Job drawing, mm, ordinate dimensions from the low corner. One solid piece. Coordinates: 2 decimals unless noted, no trailing zeros. Loops run counter-clockwise (first coordinate to the right, second up) from the corner with the lowest first, then second, coordinate; pieces in that order, holes last. Notation, with made-up numbers: M 83,53 L 139,53 A20 ccw 139,89 Z; hole C 24,54.5 d5. An arc over 180 degrees is marked long. Answer as a JSON object with one key per item and string values. Group by question number.
1. Saw through at A-A on z = 33.5. Write the cut outline in (x, y), then the cut area to 3 significant figures.
2. Drill centre lines: L1, parallel to Y at x = 80, z = 94; L2, parallel to Z at x = 13.4, y = 2.7; L3, parallel to Y at x = 30, z = 91. Where is each one in solid material? Low to high.
3. Saw through at D-D on y = 16.25. Write the cut outline in (x, z).
4. Drop flat-ended pins along their axis: pin 1 Ø12 at (x, z) = (66, 29.5) entering from +Y; pin 2 Ø7.5 at (x, y) = (80, 16.25) entering from -Z; pin 3 Ø5.5 at (x, y) = (30, 16.25) entering from -Z. Give the stop position or say it passes through.
5. Saw through at C-C on x = 13.4. Write the cut outline in (y, z).
6. Saw through at B-B on x = 80. Write the cut outline in (y, z), then the cut area to 3 significant figures.
7. Mould opens along Y. For the marked faces 1, 2 and 3 say: released by +Y, released by -Y, zero draft, split by the parting line, or undercut.
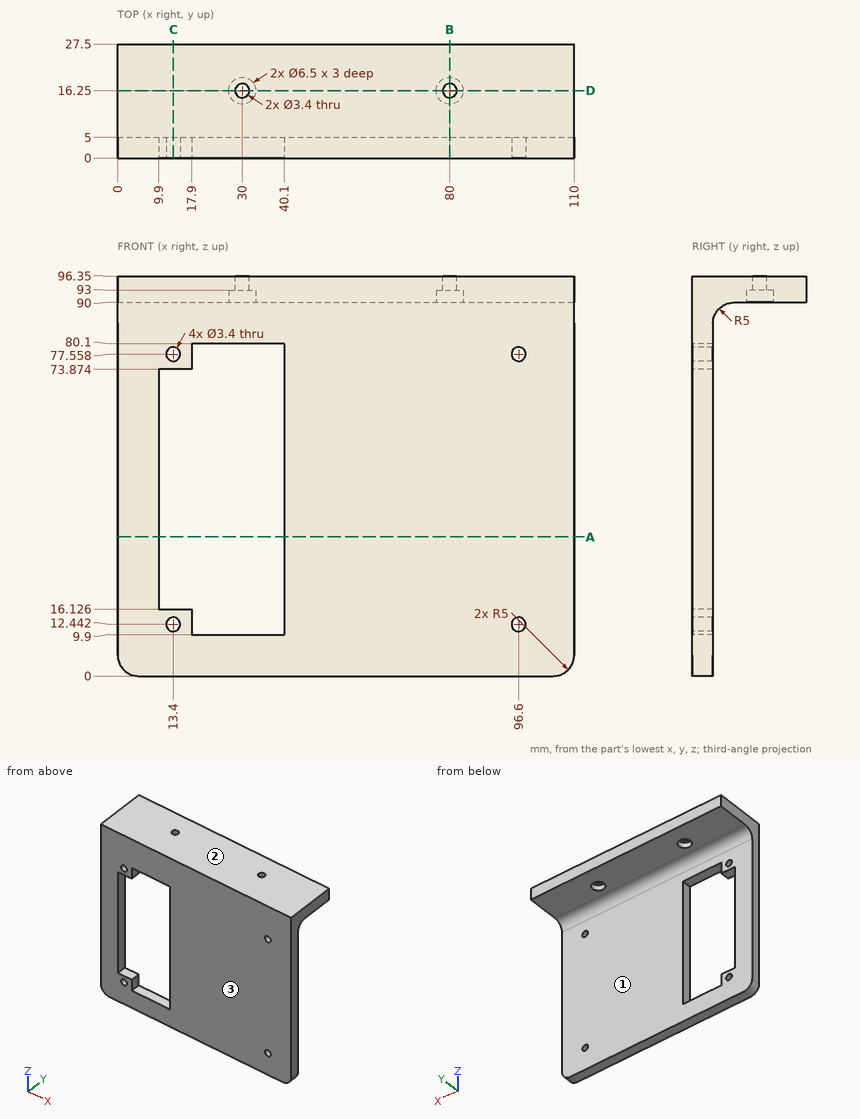
Outcome:
{
 "1": {"outline": "M 0,0 L 9.9,0 L 9.9,5 L 0,5 Z; M 40.1,0 L 110,0 L 110,5 L 40.1,5 Z", "area": "399 mm²"},
 "2": {"L1": "y = 0 to 14.55, 17.95 to 27.5", "L2": "z = 0 to 10.74, 14.14 to 16.13, 73.87 to 75.86, 79.26 to 96.35", "L3": "y = 0 to 13, 19.5 to 27.5"},
 "3": {"outline": "M 0,90 L 26.75,90 L 26.75,93 L 28.3,93 L 28.3,96.35 L 0,96.35 Z; M 31.7,93 L 33.25,93 L 33.25,90 L 76.75,90 L 76.75,93 L 78.3,93 L 78.3,96.35 L 31.7,96.35 Z; M 81.7,93 L 83.25,93 L 83.25,90 L 110,90 L 110,96.35 L 81.7,96.35 Z"},
 "4": {"pin 1": "stops at y = 5", "pin 2": "stops at z = 90", "pin 3": "stops at z = 93"},
 "5": {"outline": "M 0,0 L 5,0 L 5,10.74 L 0,10.74 Z; M 0,14.14 L 5,14.14 L 5,16.13 L 0,16.13 Z; M 0,73.87 L 5,73.87 L 5,75.86 L 0,75.86 Z; M 0,79.26 L 5,79.26 L 5,85 A5 cw 10,90 L 27.5,90 L 27.5,96.35 L 0,96.35 Z"},
 "6": {"outline": "M 0,0 L 5,0 L 5,85 A5 cw 10,90 L 13,90 L 13,93 L 14.55,93 L 14.55,96.35 L 0,96.35 Z; M 17.95,93 L 19.5,93 L 19.5,90 L 27.5,90 L 27.5,96.35 L 17.95,96.35 Z", "area": "599 mm²"},
 "7": {"face 1": "released by +Y", "face 2": "zero draft", "face 3": "released by -Y"}
}
